Autodesk Inventor part; units mm, degrees
ref_plane "YZ Plane" through (0, 0, 0) normal (1, 0, 0) x (0, 1, 0)
ref_plane "XZ Plane" through (0, 0, 0) normal (0, 1, 0) x (-1, 0, 0)
ref_plane "XY Plane" through (0, 0, 0) normal (0, 0, 1) x (1, 0, 0)
sketch "Sketch1" plane through (0, 0, 0) normal (0, 1, 0) x (-1, 0, 0)
  line L0 (-80.9017, 50) -> (80.9017, 50) construction
  line L1 (80.9017, 50) -> (80.9017, -50) construction
  line L2 (80.9017, -50) -> (-80.9017, -50) construction
  line L3 (-80.9017, -50) -> (-80.9017, 50) construction
  point P0 (0, 0)
  point P1 (0, 50)
  point P2 (80.9017, 0)
  dimension "d1" = 100
  dimension "d6" = 161.8034
sketch "Sketch2" plane through (0, 0, 0) normal (0, 0, 1) x (1, 0, 0)
  line L0 (-50, 80.9017) -> (50, 80.9017) construction
  line L1 (50, 80.9017) -> (50, -80.9017) construction
  line L2 (50, -80.9017) -> (-50, -80.9017) construction
  line L3 (-50, -80.9017) -> (-50, 80.9017) construction
  point P0 (0, 0)
  point P1 (0, 80.9017)
  point P2 (50, 0)
  dimension "d3" = 161.8034
  dimension "d7" = 100
sketch "Sketch3" plane through (0, 0, 0) normal (1, 0, 0) x (0, 1, 0)
  line L0 (-50, 80.9017) -> (50, 80.9017) construction
  line L1 (50, 80.9017) -> (50, -80.9017) construction
  line L2 (50, -80.9017) -> (-50, -80.9017) construction
  line L3 (-50, -80.9017) -> (-50, 80.9017) construction
  point P0 (0, 0)
  point P1 (50, 0)
  point P2 (0, 80.9017)
  dimension "d4" = 161.8034
  dimension "d5" = 100
sketch "Sketch7" plane through (0, 0, 0) normal (1, 0, 0) x (0, 1, 0)
  circle A0 centre (0, 0) radius 200 construction
  dimension "BallDiameter" = 400
ref_plane "Work Plane2" through (80.9017, 0, -50) normal (-0.9341724, -0.3568221, 0) x (0, 0, 1)
sketch "Sketch8" plane through (80.9017, 0, -50) normal (-0.9341724, -0.3568221, 0) x (0, 0, 1)
  line L0 (50, 86.6025) -> (0, 0) construction
  line L1 (0, 0) -> (100, 0) construction
  line L2 (100, 0) -> (50, 86.6025) construction
  line L3 (3.4641, 2) -> (50, 82.6025)
  line L4 (50, 82.6025) -> (96.5359, 2)
  line L5 (96.5359, 2) -> (3.4641, 2)
  point P0 (50, 28.8675)
  dimension "d21" = 2
  dimension "d22" = 2
  dimension "d23" = 2
extrude "Extrusion3" add sketch "Sketch8" along normal blind 2
fillet "Fillet1" radius 10 3 edges at (79.2539, 1.5115, -46.5359) (79.2539, 1.5115, 46.5359) (50.4931, 76.8082, 0)
sketch "Sketch11" plane through (80.9017, 0, -50) normal (0.9341724, 0.3568221, 0) x (0, 0, -1)
  circle A0 centre (-50, 28.8675) radius 5
  dimension "d34" = 10
hole "Hole2" at (70.6011, 26.9672, 0) direction (-0.9341724, -0.3568221, 0) diameter 10 end through all
sketch "Sketch10" plane through (80.9017, 0, -50) normal (0.9341724, 0.3568221, 0) x (0, 0, -1)
  arc A0 (-41.3397, 67.6025) -> (-58.6603, 67.6025) centre (-50, 62.6025) ccw
  circle A1 centre (-50, 62.6025) radius 1.5
  point P0 (-50, 28.8675)
  dimension "d25" = 3
hole "Hole1" at (58.5637, 58.4816, 0) direction (-0.9341724, -0.3568221, 0) diameter 3 end through all
pattern_circular "Circular Pattern1" count 3 over 360 about axis through (-28.8274, -11.0111, 0) along (0.9341724, 0.3568221, 0) of "Hole1"
equation "\"d1\" = IcoLen"
equation "\"d6\" = IcoWidth"
equation "\"d3\" = IcoWidth"
equation "\"d7\" = IcoLen"
equation "\"d4\" = IcoWidth"
equation "\"d5\" = IcoLen"
equation "\"BallDiameter\" = 2 * BallRadius"
equation "\"IcoLen\" = 100"
equation "\"IcoWidth\" = 1.61803 * IcoLen"
properties part number "Frame"
Here's how the part is built. I have some questions about the finished solid (model axes, mm). Coordinates: 2 decimals unless noted, no trailing zeros. Loops run counter-clockwise (first coordinate to the right, second up) from the corner with the lowest first, then second, coordinate; pieces in that order, holes last.
1. Imagine slicing it at B-B, the plane x = 63.5. Please give me the cut outline in (y, z).
2. Imagine slicing it at A-A, the plane y = 48. Please give me the cut outline in (x, z).
3. For P1, Ø1.5, axis at y = 17.5, z = 4, coming from the -X side; P2, Ø1, axis at y = 17, z = -1, coming from the -X side; P3, Ø8, axis at y = 30.5, z = 28, coming from the -X side; P4, Ø2, axis at x = 61.5, z = -22.5, coming from the -Y side, each with a flat end and sliding along its axis, tell me the tip position at first contact or that it passes through.
4. I need wall thicknesses on L1, parallel to X at y = 11.5, z = 15; L2, parallel to X at y = 17, z = -17; L3, parallel to Z at x = 55.5, y = 61.5. Which ranges of each line are inside material? Lowest first, please.
5. If we mould it in two halves opening along Z, with no side actions, what happens to faces 1 (the cylindrical face through (54.05, 67.46, 0.15)), 2 (the flat face through (71.145, 19.937, -0.549)), 3 (the cylindrical face through (75.347, 11.701, 30.406))? For each: pulls with the +Z half, pulls with the -Z half, needs draft (parallel to the pull), parting line crosses it, or undercut.
Taken from the geometry:
1. outline: (39.95, -22.56) - (45.56, -19.53) - (45.56, 19.53) - (39.95, 22.56) - close
2. outline: (60.43, -17.58) - (62.57, -18.02) - (62.57, 18.02) - (60.43, 17.58) - close
3. P1: stops at x = 71.79
3. P2: stops at x = 72.08
3. P3: stops at x = 65.75
3. P4: passes through
4. L1: x = 74.37 to 76.51
4. L2: x = 72.27 to 74.41
4. L3: z = -9.29 to 9.29
5. face 1: parting line crosses it
5. face 2: needs draft
5. face 3: undercut
